For this review, use the dimensioned drawing (mm, ordinates from the lowest corner) and the shaded views. A direction names the side the tool comes from. Give positions to 0.01 mm unless a question says otherwise; leave off trailing zeros. Write each loop counter-clockwise with the first axis right and the second up, starting at its lowest first coordinate (ties: lowest second). Pieces come first, ordered by that corner, then holes. Notation, with made-up numbers: M 8.25,38 L 34.25,38 A28 cw 34.25,63 Z; hole C -6,82 d6. An arc over 180 degrees is marked long. Answer in a Markdown table with one row per item.
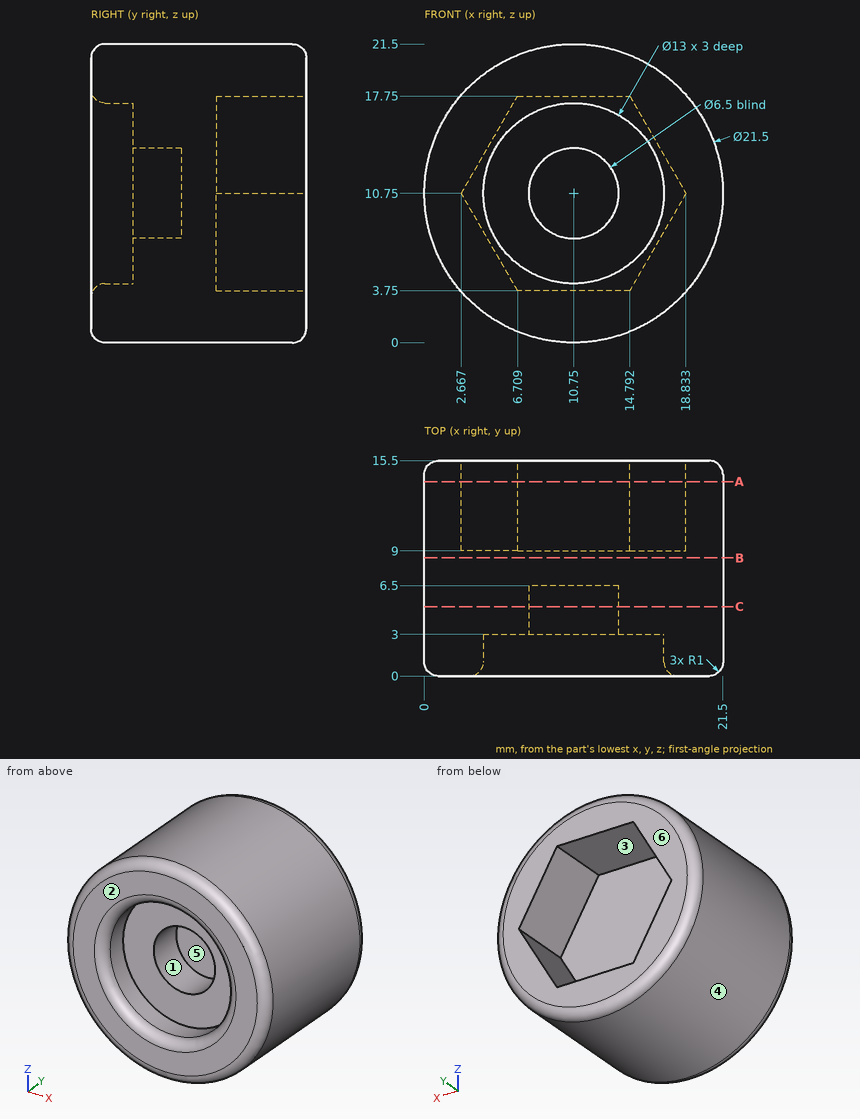
1) Add section C-C (y = 5). Write out the cut boundary in (x, z), and give its area (3 significant figures).
Geometry says:
| item | result |
|---|---|
| outline | C 10.75,10.75 d21.5; hole C 10.75,10.75 d6.5 |
| area | 330 mm^2 |
2) Add section B-B (y = 8.5). Write out the cut boundary in (x, z).
Geometry says:
| item | result |
|---|---|
| outline | C 10.75,10.75 d21.5 |
3) Insertion check: P1, Ø5, axis at x = 10, y = 11, coming from the +Z side; P2, Ø10.5, axis at x = 10.5, z = 10, coming from the -Y side; P3, Ø2, axis at x = 13.5, y = 5.5, coming from the +Z side; P4, Ø7, axis at x = 12, z = 9, coming from the +Y side. Each pin has a flat end and moves straight along its axis. Give the tip position at first contact, or say it passes through.
Geometry says:
| item | result |
|---|---|
| P1 | z = 21.5 |
| P2 | y = 3 |
| P3 | z = 21.36 |
| P4 | y = 9 |
4) For the marked faces 1, 2 and 3, list the 3-axis set-ups (+Z, -Z, +X, -X, +Y, -Y) from which the entire face can be reached by the end or side of a thin tool; tool diameter is ignored.
Geometry says:
| item | result |
|---|---|
| face 1 | -Y |
| face 2 | +Z, -Z, +X, -X, -Y |
| face 3 | +Y |
5) To check wall thickness, follow probe 1 along Z at (x, y) = (10.75, 2.1); probe 2 along Z at (x, y) = (10.75, 4.5); probe 3 along Y at (x, z) = (15, 13.25). State the ranges of each line that lie inside material, in increasing order. Write a range as [from, to].
Geometry says:
| item | result |
|---|---|
| probe 1 | [0, 4.25], [17.25, 21.5] |
| probe 2 | [0, 7.5], [14, 21.5] |
| probe 3 | [3, 9] |
6) Add section A-A (y = 14). Write out the cut boundary in (x, z), and give its area (3 significant figures).
Geometry says:
| item | result |
|---|---|
| outline | C 10.75,10.75 d21.5; hole M 2.67,10.75 L 6.71,3.75 L 14.79,3.75 L 18.83,10.75 L 14.79,17.75 L 6.71,17.75 Z |
| area | 193 mm^2 |
7) The part is to be moulded in two halves that separate along X. For the marked faces 4, 5 and 6, say which applies: released by +X, released by -X, zero draft, split by the parting line, or undercut.
Geometry says:
| item | result |
|---|---|
| face 4 | split by the parting line |
| face 5 | undercut |
| face 6 | zero draft |
